from build123d import *

# Parameters (mm, degrees)
F1_DEPTH = 7
F2_W     = 0.6
F2_H     = 3.5
F3_DEPTH = 32.5
F4_R     = 0.6
F5_R     = 1.2


with BuildPart() as f1:
    # F0 (on Right) → F1 (new body)
    with BuildSketch(Plane.YZ):
        Polygon((-46.919775, 55.204037), (-47.519775, 55.204037), (-47.519775, -16.295963), (-23.335952, 55.204037), (-23.969343, 55.204037), (-46.919775, -12.649414), align=None)
    extrude(amount=F1_DEPTH)

    # F2 (on face) → F3 (cut)
    with BuildSketch(Plane(origin=(0, -46.919775, 0), x_dir=(-1, 0, 0), z_dir=(0, 1, 0))):
        with Locations((-3.5, 53.454037)):
            Rectangle(F2_W, F2_H)
    extrude(amount=F3_DEPTH, mode=Mode.SUBTRACT)

    # F4
    f4_edges = [f1.edges().sort_by_distance(p)[0] for p in [
        (3.5, -46.919775, -12.649414),
    ]]
    fillet(f4_edges, radius=F4_R)

    # F5
    f5_edges = [f1.edges().sort_by_distance(p)[0] for p in [
        (3.5, -47.519775, -16.295963),
    ]]
    fillet(f5_edges, radius=F5_R)


solid = f1.part
Work out the finished part from the listing and answer in its coordinate system (mm). A direction names the side the tool comes from. Round coordinates to 2 decimals unless told otherwise and drop trailing zeros. Loops run counter-clockwise (first coordinate to the right, second up) from the corner with the lowest first, then second, coordinate; pieces in that order, holes last. Notation, with made-up numbers: (-1.75, -12) -> (28.25, -12) arc R12 cw to (28.25, 4) -> close; hole circle Ø8 at (-2.5, 41). An arc over 180 degrees is marked (long way). Use one line per item in the form item = value.
(1) Straight lines are drawn through the part: line 1 (Y direction, x = 2.5, z = 23); line 2 (Y direction, x = 6.5, z = 31.5); line 3 (Z direction, x = 3.75, y = -46). For each, find the intervals that lie inside material, in ascending order.
Answer list:
line_1 = -47.52 to -46.92, -34.86 to -34.23
line_2 = -47.52 to -46.92, -31.99 to -31.35
line_3 = -10.16 to -9.51
(2) Flat-ended cylindrical pins translate along their axes: P1, Ø2, axis at y = -24.5, z = 53.5, coming from the -X side; P2, Ø4, axis at x = 4.5, z = 37, coming from the +Y side. Find the tip coordinate at first contact, or state that the pin passes through.
Answer list:
P1 = 0
P2 = -28.82
(3) Find section B-B on z = 27. Give the vertices of the cut face in (x, y), then the cut area to 3 significant figures.
Answer list:
outline = (0, -47.52) -> (7, -47.52) -> (7, -46.92) -> (0, -46.92) -> close; (0, -33.51) -> (7, -33.51) -> (7, -32.88) -> (0, -32.88) -> close
area = 8.63 mm2
(4) A tool of negligible diameter and unlimited length cuts with its end or side. For faces 5 (the flat face through (3.45, -34.41, 22.46)), 6 (the flat face through (3, -46.92, 23)), from which of +Z, -Z, +X, -X, +Y, -Y can it reach the whole face along a straight path? Write none if from no direction.
Answer list:
face_5 = -Z, +X, -X, +Y
face_6 = +Z, +X, -X
(5) Find section A-A on x = 2.5. Give the vertices of the cut face in (y, z), then the cut area to 3 significant figures.
Answer list:
outline = (-47.52, -9) arc R1.2 ccw to (-45.18, -9.39) -> (-23.34, 55.2) -> (-23.97, 55.2) -> (-45.75, -9.2) arc R0.6 cw to (-46.92, -9) -> (-46.92, 55.2) -> (-47.52, 55.2) -> close
area = 80.9 mm2
(6) For a pull along X with two mould halves and no side action, classify faces 1 (the flat face through (3.451, -34.708, 23.455)), 2 (the flat face through (3.8, -24.2, 53.4)), 3 (the flat face through (7, -47.1, 22.7)), 4 (the flat face through (3.2, -24.2, 53.4)) as released by +X, released by -X, zero draft, split by the parting line, or undercut.
Answer list:
face_1 = zero draft
face_2 = undercut
face_3 = released by +X
face_4 = undercut
(7) Find section C-C on y = -33.5. Give the vertices of the cut face in (x, z), then the cut area to 3 significant figures.
Answer list:
outline = (0, 25.15) -> (7, 25.15) -> (7, 27.03) -> (0, 27.03) -> close
area = 13.1 mm2
